from build123d import *

# Parameters (mm, degrees)
SKETCH1_W           = 15
SKETCH1_H           = 15
BOSS_EXTRUDE1_DEPTH = 15
SKETCH2_R           = 6
BOSS_EXTRUDE2_DEPTH = 20
SKETCH3_R           = 6
CUT_EXTRUDE1_DEPTH  = 10
SKETCH4_R           = 3
BOSS_EXTRUDE3_DEPTH = 5


with BuildPart() as part:
    # Sketch1 → Boss-Extrude1 (new body)
    with BuildSketch(Plane.XY):
        Rectangle(SKETCH1_W, SKETCH1_H)
    extrude(amount=BOSS_EXTRUDE1_DEPTH)

    # Sketch2 → Boss-Extrude2 (add)
    with BuildSketch(Plane.XY.offset(15)):
        Circle(SKETCH2_R)
    extrude(amount=BOSS_EXTRUDE2_DEPTH)

    # Sketch3 → Cut-Extrude1 (cut)
    with BuildSketch(Plane(origin=(0, 0, 0), x_dir=(-1, 0, 0), z_dir=(0, 0, -1))):
        with Locations(Location((0, 0, 0), (0, 0, 180))):
            Circle(SKETCH3_R)
    extrude(amount=-CUT_EXTRUDE1_DEPTH, mode=Mode.SUBTRACT)

    # Sketch4 → Boss-Extrude3 (add)
    with BuildSketch(Plane.XZ.offset(7.5)):
        with Locations(Location((0, 7.5, 0), (0, 0, 270))):
            Circle(SKETCH4_R)
    extrude(amount=BOSS_EXTRUDE3_DEPTH)


solid = part.part
Read the model definition and answer for the solid it produces. Units are mm, in the model's axes. A direction names the side the tool comes from. Coordinates: 2 decimals unless noted, no trailing zeros. Order: outer loops, then holes, each group sorted by start corner. A loop starts at its lowest first (then second) coordinate and runs counter-clockwise, first axis right, second up. Notation, with made-up numbers: (64.25, 40.25) - (102.25, 40.25) arc R17 ccw to (102.25, 56.25) - close; hole circle Ø6 at (-33, -34.5). An arc over 180 degrees is marked (long way). Use one line per item in the form item = value.
(1) Straight lines are drawn through the part: L1, parallel to Y at x = 0, z = 7; L2, parallel to Z at x = -2, y = -1.5; L3, parallel to Y at x = 4, z = 7. For each, find the intervals that lie inside material, in ascending order.
Computed values:
L1 = -12.5 to -6, 6 to 7.5
L2 = 10 to 35
L3 = -7.5 to -4.47, 4.47 to 7.5
(2) Given pin 1 Ø3 at (x, y) = (-2.5, 1) entering from -Z; pin 2 Ø8 at (x, z) = (4, 23.5) entering from -Y, each flat-ended and moving along its own axis, determine where each tip first touches the part or whether it passes through.
Computed values:
pin_1 = 10
pin_2 = -6
(3) For a pull along X with two mould halves and no side action, classify faces 1 (the face through (5.723, -1.802, 4.93)), 2 (the face through (-7.5, 0, 7)), 3 (the face through (0, 0, 35)) as pulls with the +X half, pulls with the -X half, needs draft (parallel to the pull), parting line crosses it, or undercut.
Computed values:
face_1 = undercut
face_2 = pulls with the -X half
face_3 = needs draft
(4) Section D-D, the plane z = 25 is taken. Give the vertices of the cut face in (x, y), then the cut area to 3 significant figures.
Computed values:
outline = circle Ø12 at (0, 0)
area = 113 mm²
(5) Section B-B, the plane x = 0 is taken. Give the vertices of the cut face in (y, z).
Computed values:
outline = (-12.5, 4.5) - (-7.5, 4.5) - (-7.5, 0) - (-6, 0) - (-6, 10) - (6, 10) - (6, 0) - (7.5, 0) - (7.5, 15) - (6, 15) - (6, 35) - (-6, 35) - (-6, 15) - (-7.5, 15) - (-7.5, 10.5) - (-12.5, 10.5) - close
(6) Which of the six approach directions +Z, -Z, +X, -X, +Y, -Y give full straight-line access (tool end or side, diameter ignored) to faces 4 (the face through (0, -7.5, 4)), 5 (the face through (-3.44, 5.1, 15)), 6 (the face through (0, 7.5, 7)), 7 (the face through (0, 0, 10))?
Computed values:
face_4 = -Y
face_5 = +Z
face_6 = +Z, -Z, +X, -X, +Y
face_7 = -Z
(7) Section A-A, the plane y = 0 is taken. Give the vertices of the cut face in (x, z).
Computed values:
outline = (-7.5, 0) - (-6, 0) - (-6, 10) - (6, 10) - (6, 0) - (7.5, 0) - (7.5, 15) - (6, 15) - (6, 35) - (-6, 35) - (-6, 15) - (-7.5, 15) - close
(8) Section C-C, the plane z = 7.5 is taken. Give the vertices of the cut face in (x, y), then the cut area to 3 significant figures.
Computed values:
outline = (-7.5, -7.5) - (-3, -7.5) - (-3, -12.5) - (3, -12.5) - (3, -7.5) - (7.5, -7.5) - (7.5, 7.5) - (-7.5, 7.5) - close; hole circle Ø12 at (0, 0)
area = 142 mm²
